The figure shows three views and two pictorial views of one solid part (mm, origin at its lowest corner). Answer the questions. Give positions to 0.01 mm unless a question says otherwise; leave off trailing zeros. Write each loop counter-clockwise with the first axis right and the second up, starting at its lowest first coordinate (ties: lowest second). Pieces come first, ordered by that corner, then holes. Notation, with made-up numbers: (60, 13.5) -> (66, 13.5) arc R36 ccw to (66, 50.5) -> close; hole circle Ø6 at (6.25, -4.5). An arc over 180 degrees is marked (long way). Answer as CSV lines item,"result". Start each with the question number.
1. Find the intervals of material crossed by line 1 (X direction, y = 20.5, z = 1.4); line 2 (X direction, y = 3, z = 2.9); line 3 (Y direction, x = 210.5, z = 1.9), in increasing order.
2. The part is cut by section A-A, the plane x = 150. Determine the outline of the cut face in (y, z).
3. The part is cut by section D-D, the plane x = 182.5. Determine the outline of the cut face in (y, z), and give its area (3 significant figures).
4. The part is cut by section C-C, the plane z = 3.1. Determine the outline of the cut face in (x, y), and give its area (3 significant figures).
5. The part is cut by section B-B, the plane y = 20. Determine the outline of the cut face in (x, z), and give its area (3 significant figures).
6. Given pin 1 (1.5 mm diameter, centred on y = 2, z = 1.5, fed in from +X); pin 2 (2.5 mm diameter, centred on y = 2.5, z = 2.5, fed in from -X); pin 3 (1.5 mm diameter, centred on x = 77.5, z = 2, fed in from -Y), each flat-ended and moving along its own axis, determine where each tip first touches the part or whether it passes through.
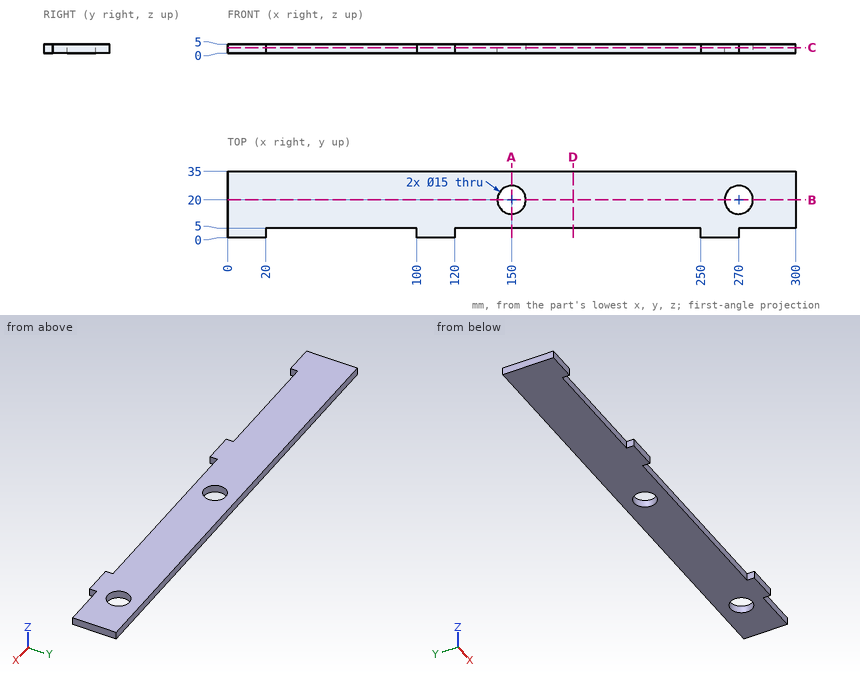
Results found:
1,line 1,"x = 0 to 142.52, 157.48 to 262.52, 277.48 to 300"
1,line 2,"x = 0 to 20, 100 to 120, 250 to 270"
1,line 3,"y = 5 to 35"
2,outline,"(5, 0) -> (12.5, 0) -> (12.5, 5) -> (5, 5) -> close; (27.5, 0) -> (35, 0) -> (35, 5) -> (27.5, 5) -> close"
3,outline,"(5, 0) -> (35, 0) -> (35, 5) -> (5, 5) -> close"
3,area,"150 mm²"
4,outline,"(0, 0) -> (20, 0) -> (20, 5) -> (100, 5) -> (100, 0) -> (120, 0) -> (120, 5) -> (250, 5) -> (250, 0) -> (270, 0) -> (270, 5) -> (300, 5) -> (300, 35) -> (0, 35) -> close; hole circle Ø15 at (150, 20); hole circle Ø15 at (270, 20)"
4,area,"8,950 mm²"
5,outline,"(0, 0) -> (142.5, 0) -> (142.5, 5) -> (0, 5) -> close; (157.5, 0) -> (262.5, 0) -> (262.5, 5) -> (157.5, 5) -> close; (277.5, 0) -> (300, 0) -> (300, 5) -> (277.5, 5) -> close"
5,area,"1,350 mm²"
6,pin 1,"stops at x = 270"
6,pin 2,"stops at x = 0"
6,pin 3,"stops at y = 5"
